Answer from the drawing. Dimensions are ordinates in mm from the lowest x, y and z of the part. A direction names the side the tool comes from. Round coordinates to 2 decimals unless told otherwise and drop trailing zeros. Order: outer loops, then holes, each group sorted by start corner. A loop starts at its lowest first (then second) coordinate and runs counter-clockwise, first axis right, second up. Notation, with made-up numbers: (-27.5, -26.5) -> (1.5, -26.5) arc R17 ccw to (1.5, 2.5) -> close; hole circle Ø1 at (-36, 31.25). An arc over 180 degrees is marked (long way). Use a Markdown table: item, result. Add a question column.
1. Consider L1, parallel to Y at x = 33.5, z = 5.5; L2, parallel to X at y = 19, z = 5.25 (3 decimals); L3, parallel to X at y = 13.5, z = 11.75. Determine where each line is inside the solid, lowest interval first. Write a range as [from, to].
2. Given pin 1 (3 mm diameter, centred on x = 219.5, z = 1.5, fed in from +Y); pin 2 (6 mm diameter, centred on x = 21, z = 4, fed in from -Y); pin 3 (1 mm diameter, centred on x = 202.5, y = 25, fed in from -Z); pin 4 (12 mm diameter, centred on x = 48, y = 23, fed in from -Z), each flat-ended and moving along its own axis, determine where each tip first touches the part or whether it passes through.
3. For the marked faces 1 and 2, determine the directions among +Z, -Z, +X, -X, +Y, -Y from which every point of the face is accessible in a straight line to the end or side of a thin tool.
4. Section A-A, the plane x = 196 is taken. Give the vertices of the cut face in (y, z).
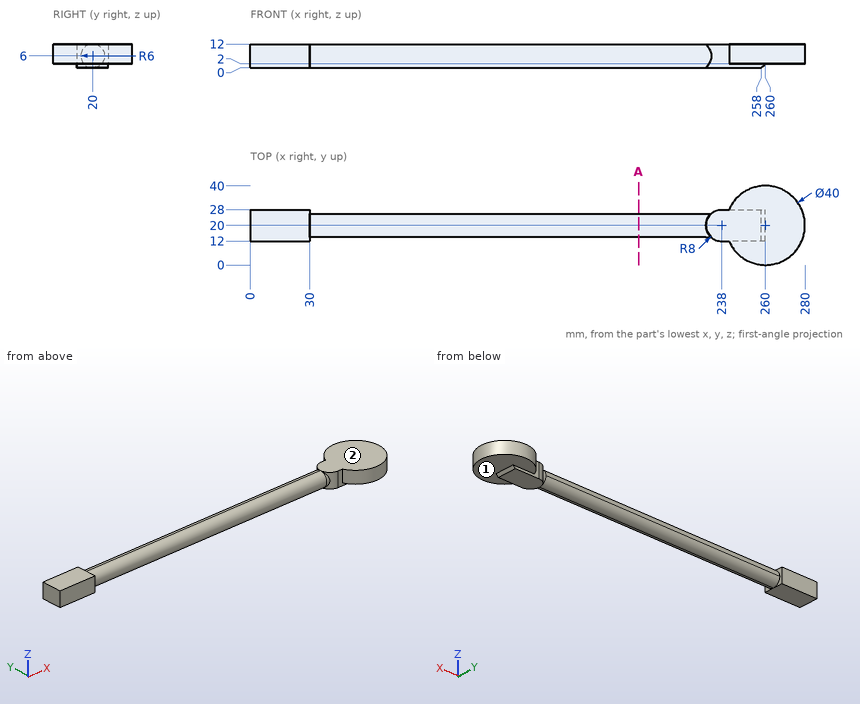
Verdict:
| question | item | result |
|---|---|---|
| 1 | L1 | y = [14.02, 25.98] |
| 1 | L2 | x = [0, 279.975] |
| 1 | L3 | x = [0, 30], [233.34, 278.91] |
| 2 | pin 1 | stops at y = 25.2 |
| 2 | pin 2 | stops at y = 12 |
| 2 | pin 3 | stops at z = 2.03 |
| 2 | pin 4 | stops at z = 0 |
| 3 | face 1 | -Z, +X |
| 3 | face 2 | +Z, +X, -X, +Y, -Y |
| 4 | outline | circle Ø12 at (20, 6) |
